For this review, use the dimensioned drawing (mm, ordinates from the lowest corner) and the shaded views. Coordinates: 2 decimals unless noted, no trailing zeros. Write each loop counter-clockwise with the first axis right and the second up, starting at its lowest first coordinate (ties: lowest second). Pieces come first, ordered by that corner, then holes. Notation, with made-up numbers: (-5.5, 23.25) - (38.5, 23.25) arc R23 ccw to (38.5, 47.25) - close; hole circle Ø9 at (68, -36). An arc over 180 degrees is marked (long way). Put each result on its own line as item: value.
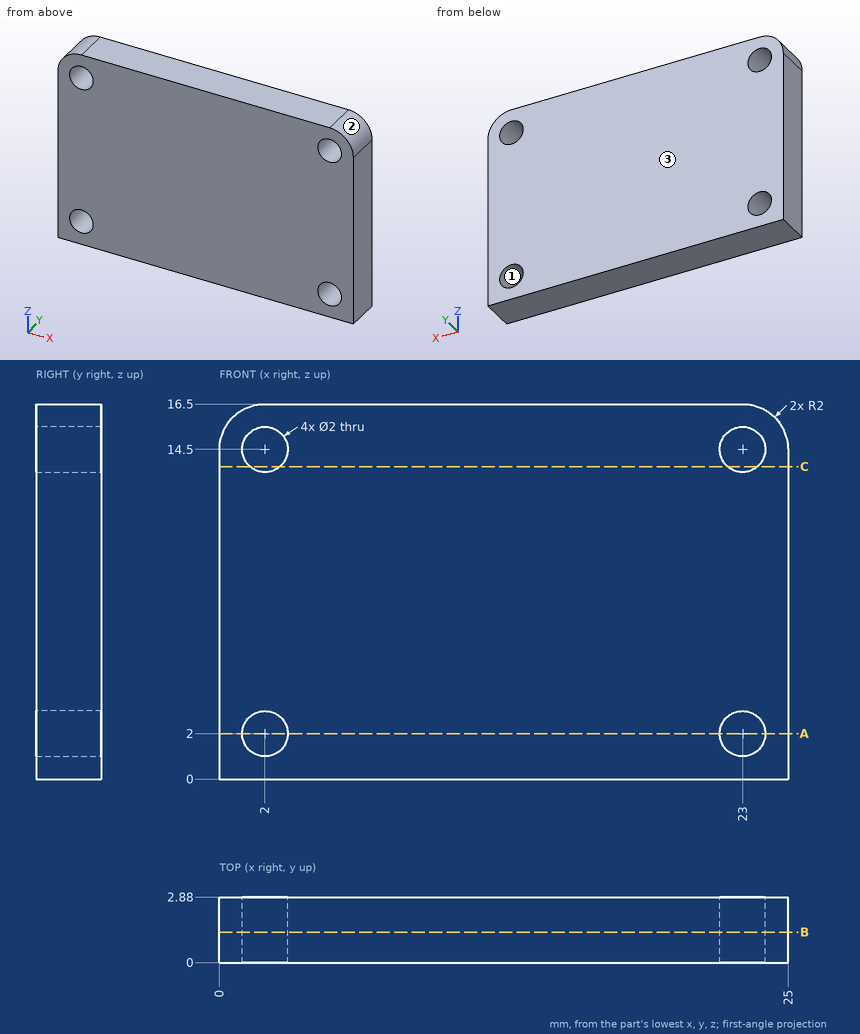
1. To check wall thickness, follow probe 1 along X at (y, z) = (1.85, 14.5); probe 2 along Z at (x, y) = (23.25, 1). State the ranges of each line that lie inside material, in increasing order.
Determined:
probe 1: x = 0 to 1, 3 to 22, 24 to 25
probe 2: z = 0 to 1.03, 2.97 to 13.53, 15.47 to 16.48
2. Consider section A-A on z = 2. State the section outline as (x, y) points, plus the area to 3 significant figures.
Determined:
outline: (0, 0) - (1, 0) - (1, 2.88) - (0, 2.88) - close; (3, 0) - (22, 0) - (22, 2.88) - (3, 2.88) - close; (24, 0) - (25, 0) - (25, 2.88) - (24, 2.88) - close
area: 60.5 mm^2
3. The part is to be moulded in two halves that separate along X. For the marked faces 1, 2 and 3, say which applies: +X half, -X half, draft (parallel to the pull), parting line (faces both ways), or undercut.
Determined:
face 1: undercut
face 2: +X half
face 3: draft
4. Consider section C-C on z = 13.75. State the section outline as (x, y) points, plus the area to 3 significant figures.
Determined:
outline: (0, 0) - (1.34, 0) - (1.34, 2.88) - (0, 2.88) - close; (2.66, 0) - (22.34, 0) - (22.34, 2.88) - (2.66, 2.88) - close; (23.66, 0) - (25, 0) - (25, 2.88) - (23.66, 2.88) - close
area: 64.4 mm^2
5. Consider section B-B on y = 1.35. State the section outline as (x, z) points.
Determined:
outline: (0, 0) - (25, 0) - (25, 14.5) arc R2 ccw to (23, 16.5) - (2, 16.5) arc R2 ccw to (0, 14.5) - close; hole circle Ø2 at (2, 2); hole circle Ø2 at (2, 14.5); hole circle Ø2 at (23, 2); hole circle Ø2 at (23, 14.5)
6. For pin 1 Ø3 at (x, z) = (23, 2) entering from +Y, flat-tipped, find the tip position at first contact; note if it passes through.
Determined:
pin 1: stops at y = 2.88
